Verification items for the finished model (mm, model axes). A direction names the side the tool comes from. Coordinates: 2 decimals unless noted, no trailing zeros. Order: outer loops, then holes, each group sorted by start corner. A loop starts at its lowest first (then second) coordinate and runs counter-clockwise, first axis right, second up. Notation, with made-up numbers: M 87.5,-8 L 142.5,-8 A28 ccw 142.5,17 Z; hole C 21,77 d3. An arc over 180 degrees is marked long. Return JSON: item names as keys, results as strings. Group by question number.
Q1. Access from +Z, -Z, +X, -X, +Y, -Y to the whole of each face (thin tool, end or side, straight path). Record for faces 4 (the face through (-29.062, 20, 24)), 5 (the face through (9, -5.244, 24)), 6 (the face through (12, -10, 22.5)).
Q2. Thickness scan on probe 1 along Z at (x, y) = (-37.5, 5.5); probe 2 along X at (y, z) = (0.5, 1.25); probe 3 along X at (y, z) = (-13.5, 14.75). Record the ranges inside material, lowest first.
Q3. Section check B-B, the plane x = 2. Enter the section's corners in (y, z), then the cut area to 3 significant figures.
Q4. Mould release check, pull along X, two halves, no side actions. Record for faces 1 (the face through (-39, 24, 22.5)), 2 (the face through (-29.062, 20, 1)), 3 (the face through (22.937, -10.134, 23.732)): pulls with the +X half, pulls with the -X half, needs draft (parallel to the pull), parting line crosses it, or undercut.
Q5. Section check C-C, the plane x = -41.5. Enter the section's corners in (y, z).
Q6. Section check A-A, the plane y = 31. Enter the section's corners in (x, z), then the cut area to 3 significant figures.
Q7. Section check D-D, the plane z = 8. Enter the section's corners in (x, y).
Q8. Go/stop test with flat-tipped pins: pin 1 Ø10 at (x, z) = (-4, 22) entering from +Y; pin 2 Ø5 at (y, z) = (26, 21) entering from +X; pin 3 Ø3 at (x, y) = (-5.5, 7.5) entering from -Z; pin 4 Ø7.5 at (x, z) = (-29, 12.5) entering from +Y. Record where each tip stops, or that it passes through.
from build123d import *

# Parameters (mm, degrees)
BOSS_EXTRUDE1_DEPTH     = 25
CUT_EXTRUDE2_DEPTH      = 77.188110548
CUT_EXTRUDE2_DEPTH_BACK = 77.188110548
SKETCH3_W               = 20
SKETCH3_H               = 56.795841011
SKETCH4_R               = 5
CUT_EXTRUDE3_DEPTH      = 75.213706527
SKETCH5_R               = 2.5
CUT_EXTRUDE4_DEPTH      = 75.213706527
CUT_EXTRUDE5_REACH      = 79.827
SKETCH7_W               = 25.650683803
SKETCH7_H               = 20
SKETCH8_R               = 2.5
CUT_EXTRUDE6_DEPTH      = 75.213706527


with BuildPart() as part:
    # Sketch1 → Boss-Extrude1 (new body)
    with BuildSketch(Plane.XY):
        with BuildLine():
            Line((-49.061655574, -20.24431501), (-49.061655574, 39.75568499))
            ThreePointArc((-49.061655574, 39.75568499), (-39.061655574, 49.75568499), (-29.061655574, 39.75568499))
            Line((-29.061655574, 39.75568499), (-29.061655574, -0.24431501))
            Line((-29.061655574, -0.24431501), (-9.061655574, -0.24431501))
            Line((-9.061655574, -0.24431501), (-9.061655574, 9.75568499))
            ThreePointArc((-9.061655574, 9.75568499), (-4.061655574, 14.75568499), (0.938344426, 9.75568499))
            Line((0.938344426, 9.75568499), (0.938344426, -5.24431501))
            Line((0.938344426, -5.24431501), (17.938344426, -5.24431501))
            ThreePointArc((17.938344426, -5.24431501), (22.938344426, -10.24431501), (17.938344426, -15.24431501))
            Line((17.938344426, -15.24431501), (0.938344426, -15.24431501))
            Line((0.938344426, -15.24431501), (0.938344426, -20.24431501))
            Line((0.938344426, -20.24431501), (-49.061655574, -20.24431501))
        make_face()
    extrude(amount=BOSS_EXTRUDE1_DEPTH)

    # Sketch3 → Cut-Extrude2 (cut, two sides: drawn at the far end of the back side and taken through both)
    with BuildSketch(Plane(origin=(-29.061655574, 0, 0), x_dir=(0, 0, -1), z_dir=(1, 0, 0)).offset(-CUT_EXTRUDE2_DEPTH_BACK)):
        with Locations((-12.5, 28.153605496)):
            Rectangle(SKETCH3_W, SKETCH3_H)
    extrude(amount=CUT_EXTRUDE2_DEPTH + CUT_EXTRUDE2_DEPTH_BACK, mode=Mode.SUBTRACT)

    # Sketch4 → Cut-Extrude3 (cut, through all)
    with BuildSketch(Plane.XY.offset(25)):
        with Locations((-39.061655574, 39.75568499)):
            Circle(SKETCH4_R)
    extrude(amount=-CUT_EXTRUDE3_DEPTH, mode=Mode.SUBTRACT)

    # Sketch5 → Cut-Extrude4 (cut, through all)
    with BuildSketch(Plane.XY.offset(25)):
        with Locations((-4.061655574, 9.75568499)):
            Circle(SKETCH5_R)
    extrude(amount=-CUT_EXTRUDE4_DEPTH, mode=Mode.SUBTRACT)

    # Sketch7 → Cut-Extrude5 (cut, up to next)
    with BuildSketch(Plane(origin=(0, -5.24431501, 0), x_dir=(1, 0, 0), z_dir=(0, 1, 0)), mode=Mode.PRIVATE) as cut_extrude5_sk1:
        with Locations((13.763686328, -12.5)):
            Rectangle(SKETCH7_W, SKETCH7_H)
    cut_extrude5_tool1 = extrude(cut_extrude5_sk1.sketch, amount=-CUT_EXTRUDE5_REACH, mode=Mode.PRIVATE) & part.part
    add(cut_extrude5_tool1.solids().sort_by_distance((13.763686, -5.244315, 12.5))[0], mode=Mode.SUBTRACT)

    # Sketch8 → Cut-Extrude6 (cut, through all)
    with BuildSketch(Plane.XY.offset(25)):
        with Locations((17.938344426, -10.24431501)):
            Circle(SKETCH8_R)
    extrude(amount=-CUT_EXTRUDE6_DEPTH, mode=Mode.SUBTRACT)


solid = part.part
Numbers:
{
 "1": {"face 4": "+Z, -Z, +Y", "face 5": "+Z, -Z, +X, +Y", "face 6": "+X, +Y, -Y"},
 "2": {"probe 1": "z = 0 to 2.5, 22.5 to 25", "probe 2": "x = -49.06 to -29.06, -9.06 to 0.94", "probe 3": "x = -49.06 to 0.94"},
 "3": {"outline": "M -15.24,0 L -5.24,0 L -5.24,2.5 L -15.24,2.5 Z; M -15.24,22.5 L -5.24,22.5 L -5.24,25 L -15.24,25 Z", "area": "50.0 mm2"},
 "4": {"face 1": "needs draft", "face 2": "undercut", "face 3": "pulls with the +X half"},
 "5": {"outline": "M -20.24,0 L 35.39,0 L 35.39,2.5 L -0.24,2.5 L -0.24,22.5 L 35.39,22.5 L 35.39,25 L -20.24,25 Z; M 44.12,0 L 49.45,0 L 49.45,2.5 L 44.12,2.5 Z; M 44.12,22.5 L 49.45,22.5 L 49.45,25 L 44.12,25 Z"},
 "6": {"outline": "M -49.06,0 L -29.06,0 L -29.06,2.5 L -49.06,2.5 Z; M -49.06,22.5 L -29.06,22.5 L -29.06,25 L -49.06,25 Z", "area": "100 mm2"},
 "7": {"outline": "M -49.06,-20.24 L 0.94,-20.24 L 0.94,-0.24 L -49.06,-0.24 Z"},
 "8": {"pin 1": "stops at y = 14.76", "pin 2": "stops at x = -29.06", "pin 3": "stops at z = 0", "pin 4": "stops at y = -0.24"}
}
